Design review of the part built by this model. Coordinates are the model's own, in mm. Coordinates: 2 decimals unless noted, no trailing zeros. Loops run counter-clockwise (first coordinate to the right, second up) from the corner with the lowest first, then second, coordinate; pieces in that order, holes last. Notation, with made-up numbers: (-31.5, -31) -> (10.5, -31) arc R26 ccw to (10.5, 0) -> close; hole circle Ø1 at (80.5, 25.25). An arc over 180 degrees is marked (long way). One line per item, written item: value. Start each with the question number.
1. Add section A-A on x = 0. Write out the cut boundary in (y, z), plus the area to 3 significant figures.
2. Draft analysis for pull direction Y (two halves, no side actions). For faces 1 (the flat face through (8.2, 0.3, 5.8)), 2 (the cylindrical face through (-17.24, 17.14, 2.94)), 3 (the cylindrical face through (-1.73, -7.81, 2.94)), state which applies: pulls with the +Y half, pulls with the -Y half, needs draft (parallel to the pull), parting line crosses it, or undercut.
3. For probe 1 along Y at (x, z) = (0, 3); probe 2 along Y at (x, z) = (-13, 1.5); probe 3 along X at (y, z) = (-4, 1), list the stretches that pass through material, from the lowest coordinate up.
4. Add section C-C on x = 4. Write out the cut boundary in (y, z), plus the area to 3 significant figures.
```python
from build123d import *

# Parameters (mm, degrees)
SKETCH1_W           = 38.1
SKETCH1_H           = 38.1
BOSS_EXTRUDE1_DEPTH = 5.8
SKETCH2_R           = 0.79375
CUT_EXTRUDE1_DEPTH  = 28.558029683
SKETCH3_R           = 8
CUT_EXTRUDE2_DEPTH  = 12.7
FILLET1_R           = 6.35


with BuildPart() as part:
    # Sketch1 → Boss-Extrude1 (new body)
    with BuildSketch(Plane.XY):
        Rectangle(SKETCH1_W, SKETCH1_H)
    extrude(amount=BOSS_EXTRUDE1_DEPTH)

    # Sketch2 → Cut-Extrude1 (cut, through all)
    with BuildSketch(Plane.XY.offset(5.8)):
        with Locations((0, 15.875)):
            Circle(SKETCH2_R)
        with Locations((15.875, 0)):
            Circle(SKETCH2_R)
        with Locations((0, -15.875)):
            Circle(SKETCH2_R)
        with Locations((-15.875, 0)):
            Circle(SKETCH2_R)
    extrude(amount=-CUT_EXTRUDE1_DEPTH, mode=Mode.SUBTRACT)

    # Sketch3 → Cut-Extrude2 (cut)
    with BuildSketch(Plane.XY.offset(5.8)):
        Circle(SKETCH3_R)
    extrude(amount=-CUT_EXTRUDE2_DEPTH, mode=Mode.SUBTRACT)

    # Fillet1
    fillet1_edges = [part.edges().sort_by_distance(p)[0] for p in [
        (19.05, -19.05, 2.9),
        (-19.05, -19.05, 2.9),
        (-19.05, 19.05, 2.9),
        (19.05, 19.05, 2.9),
    ]]
    fillet(fillet1_edges, radius=FILLET1_R)


solid = part.part
```
Worked answers:
1. outline: (-19.05, 0) -> (-16.67, 0) -> (-16.67, 5.8) -> (-19.05, 5.8) -> close; (-15.08, 0) -> (-8, 0) -> (-8, 5.8) -> (-15.08, 5.8) -> close; (8, 0) -> (15.08, 0) -> (15.08, 5.8) -> (8, 5.8) -> close; (16.67, 0) -> (19.05, 0) -> (19.05, 5.8) -> (16.67, 5.8) -> close
1. area: 110 mm²
2. face 1: needs draft
2. face 2: pulls with the +Y half
2. face 3: undercut
3. probe 1: y = -19.05 to -16.67, -15.08 to -8, 8 to 15.08, 16.67 to 19.05
3. probe 2: y = -19.04 to 19.04
3. probe 3: x = -19.05 to -6.93, 6.93 to 19.05
4. outline: (-19.05, 0) -> (-6.93, 0) -> (-6.93, 5.8) -> (-19.05, 5.8) -> close; (6.93, 0) -> (19.05, 0) -> (19.05, 5.8) -> (6.93, 5.8) -> close
4. area: 141 mm²
